Geometry check sheet. Reference: drawing and pictorial views, mm from the part's lowest x, y, z. Give positions to 0.01 mm unless a question says otherwise; leave off trailing zeros. Order: outer loops, then holes, each group sorted by start corner. A loop starts at its lowest first (then second) coordinate and runs counter-clockwise, first axis right, second up.
Item 1: Sectioned sample at B-B on z = 112.5. Record the boundary of the cut face in (x, y), and give its area (3 significant figures).
Item 2: Material ranges on line 1 along Y through (x, z) = (31, 210); line 2 along Z through (x, y) = (4, 10), recorded low to high.
Item 3: Sectioned sample at C-C on x = 24. Record the boundary of the cut face in (y, z), and give its area (3 significant figures).
Item 4: Sectioned sample at A-A on y = 3. Record the boundary of the cut face in (x, z), and give its area (3 significant figures).
Item 5: Gauge pin test, flat ends, axial feed: P1, Ø5, axis at x = 2.5, y = 16, coming from the +Z side; P2, Ø12, axis at x = 29.5, z = 125, coming from the +Y side; P3, Ø7, axis at y = 4.5, z = 261.5, coming from the -X side. Record the tip position at first contact, or that the pin passes through.
Item 6: Sectioned sample at D-D on y = 30.5. Record the boundary of the cut face in (x, z), and give its area (3 significant figures).
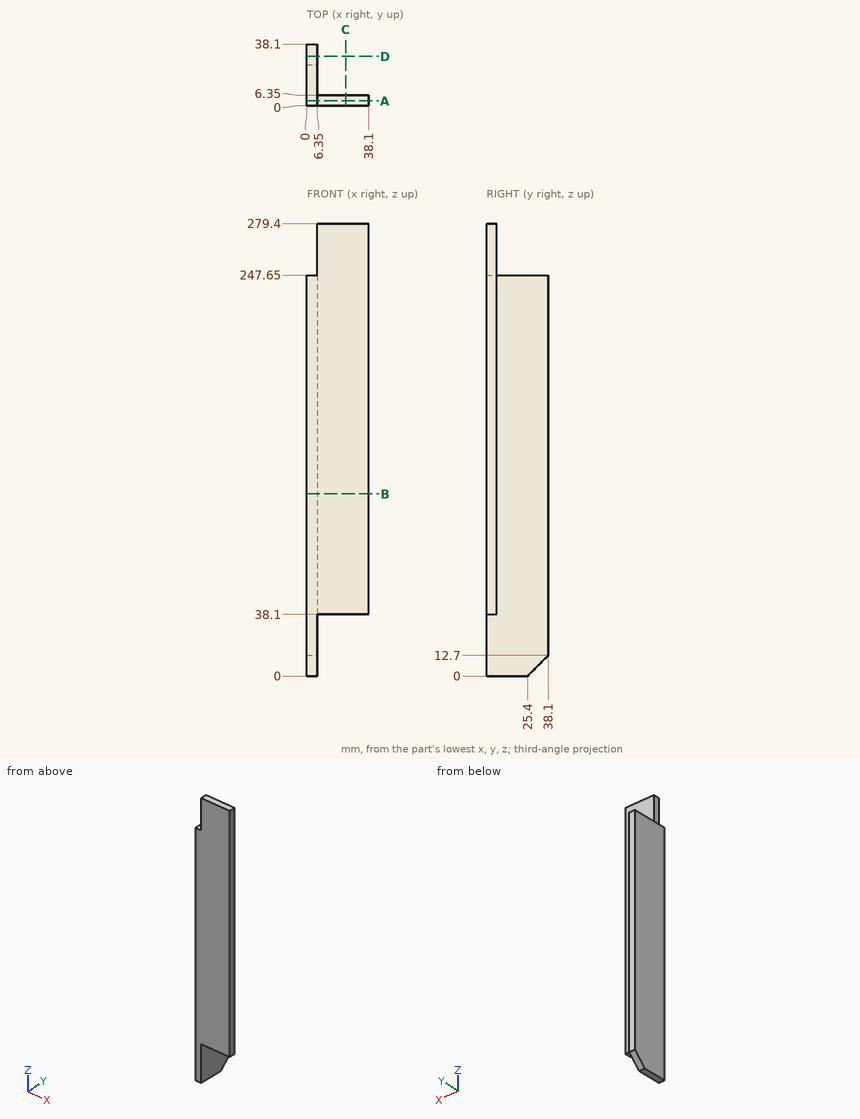
Report:
1. outline: (0, 0) - (38.1, 0) - (38.1, 6.35) - (6.35, 6.35) - (6.35, 38.1) - (0, 38.1) - close
1. area: 444 mm2
2. line 1: y = 0 to 6.35
2. line 2: z = 0 to 247.65
3. outline: (0, 38.1) - (6.35, 38.1) - (6.35, 279.4) - (0, 279.4) - close
3. area: 1,530 mm2
4. outline: (0, 0) - (6.35, 0) - (6.35, 38.1) - (38.1, 38.1) - (38.1, 279.4) - (6.35, 279.4) - (6.35, 247.65) - (0, 247.65) - close
4. area: 9,230 mm2
5. P1: stops at z = 247.65
5. P2: stops at y = 6.35
5. P3: stops at x = 6.35
6. outline: (0, 5.1) - (6.35, 5.1) - (6.35, 247.65) - (0, 247.65) - close
6. area: 1,540 mm2
